Model file for the job. Use its own axes, mm. Round coordinates to 2 decimals unless told otherwise and drop trailing zeros. Loops run counter-clockwise (first coordinate to the right, second up) from the corner with the lowest first, then second, coordinate; pieces in that order, holes last. Notation, with made-up numbers: (70, 77.5) -> (90, 77.5) arc R15 cw to (90, 84.5) -> close; hole circle Ø7 at (82.5, 52.25). An arc over 180 degrees is marked (long way). Use a Markdown table: item, result.
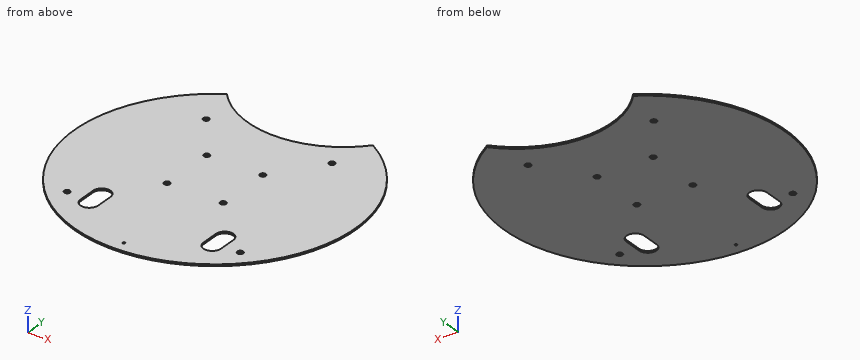
Autodesk Fusion 360 part; units mm, degrees
sketch "Esboço1" plane through (0, 0, 0) normal (0, 0, 1) x (1, 0, 0)
  circle A0 centre (0, 0) radius 240
  line L0 (48, -48) -> (-48, -48)
  line L1 (-48, -48) -> (-48, 48)
  line L2 (-48, 48) -> (48, 48)
  line L3 (48, 48) -> (48, -48)
  line L4 (48, -48) -> (-48, 48) construction
  line L5 (-48, -48) -> (48, 48) construction
  circle A1 centre (-48, 48) radius 5
  circle A2 centre (-48, -48) radius 5
  circle A3 centre (48, 48) radius 5
  circle A4 centre (48, -48) radius 5
  line L6 (105, -110) -> (105, -170)
  line L7 (90, -125) -> (90, -155)
  line L8 (120, -125) -> (120, -155)
  arc A5 (120, -125) -> (90, -125) centre (105, -125) ccw
  arc A6 (90, -155) -> (120, -155) centre (105, -155) ccw
  circle A7 centre (148, -148) radius 5
  line L9 (-125, 204.878) -> (125, 204.878)
  circle A8 centre (0, 311.043) radius 164
  circle A9 centre (107.5, 130.5) radius 5
  line L10 (-40, 115) -> (40, 115)
  line L11 (-40, 115) -> (-40, 151.9958)
  line L12 (40, 115) -> (40, 151.9958)
  line L13 (0, 1.75) -> (0, 22.5)
  line L14 (-120, -125) -> (-120, -155)
  arc A10 (-90, -125) -> (-120, -125) centre (-105, -125) ccw
  line L15 (-90, -125) -> (-90, -155)
  arc A11 (-120, -155) -> (-90, -155) centre (-105, -155) ccw
  circle A12 centre (-148, -148) radius 5
  circle A13 centre (-107.5, 130.5) radius 5
  circle A14 centre (0, -220) radius 2
  point P0 (105, -110)
  point P1 (0, 115)
  dimension "d1" = 480
  dimension "d2" = 96
  dimension "d3" = 96
  dimension "d4" = 10
  dimension "d5" = 10
  dimension "d6" = 10
  dimension "d7" = 10
  dimension "d8" = 110
  dimension "d9" = 105
  dimension "d10" = 30
  dimension "d11" = 60
  dimension "d12" = 30
  dimension "d13" = 10
  dimension "d14" = 148
  dimension "d15" = 148
  dimension "d16" = 250
  dimension "d17" = 328
  dimension "d18" = 10
  dimension "d19" = 130.5
  dimension "d20" = 107.5
  dimension "d21" = 115
  dimension "d22" = 80
  dimension "d23" = 4
  dimension "d24" = 220
extrude "Extrusão1" add sketch "Esboço1" along normal blind 3 contours A0 A8 L10 L11 L12 | A8 L10 L11 L12 | L0 L1 L2 L3 A1 A2 A3 A4
equation "d12 = d10"
equation "d17 = ( 164 * 2 ) * 1 mm"
equation "d24 = d1 / 2 - 20 mm"
Q1. Band-saw the part on B-B, the plane x = -209.5. Give the cut face in (y, z).
Results list:
| item | result |
|---|---|
| outline | (-117.09, 0) -> (117.09, 0) -> (117.09, 3) -> (-117.09, 3) -> close |
Q2. Flat gauge pins, fed straight in: pin 1 (0.9 mm diameter, centred on y = -141, z = 1.5, fed in from -X); pin 2 (5 mm diameter, centred on x = 0, y = -220, fed in from -Z); pin 3 (1.5 mm diameter, centred on y = -136, z = 1.5, fed in from +X); pin 4 (6 mm diameter, centred on x = 48, y = 48, fed in from -Z). Where does each tip first touch, or does it go through?
Results list:
| item | result |
|---|---|
| pin 1 | stops at x = -194.54 |
| pin 2 | stops at z = 0 |
| pin 3 | stops at x = 198.26 |
| pin 4 | passes through |
Q3. Band-saw the part on A-A, the plane z = 2.55. Give the number of separate pieces and of enclosed holes in the cut face, plus the area to 3 significant figures.
Results list:
| item | result |
|---|---|
| separate pieces | 1 |
| enclosed holes | 11 |
| area | 161,000 mm² |
Q4. Band-saw the part on C-C, the plane x = -19. Give the cut face in (y, z), plus the area to 3 significant figures.
Results list:
| item | result |
|---|---|
| outline | (-239.25, 0) -> (148.15, 0) -> (148.15, 3) -> (-239.25, 3) -> close |
| area | 1,160 mm² |
Q5. Drill centre lines: L1, parallel to Y at x = 107.5, z = 1.5; L2, parallel to X at y = -135.5, z = 1.85; L3, parallel to X at y = -133, z = 1.2. Where is each one in solid material? Low to high. Write a range as from..to.
Results list:
| item | result |
|---|---|
| L1 | y = -214.58..-169.79, -110.21..125.5, 135.5..187.19 |
| L2 | x = -198.09..-120, -90..90, 120..198.09 |
| L3 | x = -199.78..-120, -90..90, 120..199.78 |
